```python
from build123d import *

# Parameters (mm, degrees)
STEM_START                = 6.825155764
STEM_OTHER_SIDE_OUTLINE_W = 12.827
STEM_OTHER_SIDE_OUTLINE_H = 3.302
STEM_OTHER_SIDE_OUTLINE_R = 3.81
STEM_OTHER_SIDE_DEPTH     = 3.175
SKETCH2_R                 = 1.5875
CUT_EXTRUDE1_DEPTH        = 3.175
FILLET1_R                 = 8.89
FILLET2_R                 = 8.89


# Read off the part's stored shape, not the designer's step: Stem Other Side
with BuildPart() as part:
    # Stem Other Side outline → Stem Other Side (new body)
    with BuildSketch(Plane(origin=(0, 0, 0), x_dir=(1, 0, 0), z_dir=(0, 1, 0)).offset(STEM_START)):
        with BuildLine():
            Line((-15.619811821, 34.159467437), (-16.889811821, 34.159467437))
            ThreePointArc((-16.889811821, 34.159467437), (-23.175991106, 31.555646722), (-25.779811821, 25.269467437))
            Line((-25.779811821, 25.269467437), (-25.779811821, -42.040532563))
            Line((-25.779811821, -42.040532563), (-6.729811821, -42.040532563))
            Line((-6.729811821, -42.040532563), (-6.729811821, 25.269467437))
            ThreePointArc((-6.729811821, 25.269467437), (-9.333632536, 31.555646722), (-15.619811821, 34.159467437))
        make_face()
        with Locations((-16.254811821, -11.941532563)):
            Rectangle(STEM_OTHER_SIDE_OUTLINE_W, STEM_OTHER_SIDE_OUTLINE_H, mode=Mode.SUBTRACT)
        with Locations((-16.254811821, 21.459467437)):
            Circle(STEM_OTHER_SIDE_OUTLINE_R, mode=Mode.SUBTRACT)
    extrude(amount=STEM_OTHER_SIDE_DEPTH)

    # Sketch2 → Cut-Extrude1 (cut)
    with BuildSketch(Plane(origin=(0, 10.000155764, 0), x_dir=(1, 0, 0), z_dir=(0, 1, 0))):
        with Locations(Location((-16.254811821, -29.340532563, 0), (0, 0, 270))):
            Circle(SKETCH2_R)
    extrude(amount=-CUT_EXTRUDE1_DEPTH, mode=Mode.SUBTRACT)

    # Fillet1
    fillet1_edges = [part.edges().sort_by_distance(p)[0] for p in [
        (-6.729811821, 8.412655764, 42.040532563),
    ]]
    fillet(fillet1_edges, radius=FILLET1_R)

    # Fillet2
    fillet2_edges = [part.edges().sort_by_distance(p)[0] for p in [
        (-25.779811821, 8.412655764, 42.040532563),
    ]]
    fillet(fillet2_edges, radius=FILLET2_R)


solid = part.part
```
Can you work these out from the model? Positions are in its coordinate system, mm. A direction names the side the tool comes from. Round coordinates to 2 decimals unless told otherwise and drop trailing zeros. Loops run counter-clockwise (first coordinate to the right, second up) from the corner with the lowest first, then second, coordinate; pieces in that order, holes last.
Item 1: Please list where these lines run through material, in increasing order: L1, parallel to Z at x = -18.25, y = 8.4; L2, parallel to Z at x = -17.5, y = 8.7; L3, parallel to X at y = 8.7, z = -22.5.
Item 2: Suppose I cut it at C-C, the plane z = -27.5. Write out the boundary of the cut face in (x, y).
Item 3: Which directions (+Z, -Z, +X, -X, +Y, -Y) give clear straight access to the entire face, cutting with the end or side of a thin tool? Please do faces 4 (the flat face through (-16, 8, 10.291)), 5 (the flat face through (-16, 10, 3)).
Item 4: Will this pin go through, and if not, where does the flat tip stop? pin 1 Ø5 at (x, z) = (-16.25, 29.34) entering from +Y.
Item 5: Suppose I cut it at A-A, the plane y = 9.3. Write out the boundary of the cut face in (x, z) (1 decimal), then the cut area to 3 significant figures.
Item 6: Suppose I cut it at B-B, the plane z = 35.5. Write out the boundary of the cut face in (x, y).
Item 7: If we mould it in two halves opening along Z, with no side actions, what happens to faces 1 (the cylindrical face through (-9.265, 8.435, 39.367)), 2 (the flat face through (-25.78, 8, 4)), 3 (the flat face through (-9.841, 8, 12))? For each: +Z half, -Z half, draft (parallel to the pull), parting line (faces both ways), or undercut.
Reported:
1. L1: z = -34.05 to -24.71, -18.21 to 10.29, 13.59 to 41.94
1. L2: z = -34.14 to -25.06, -17.86 to 10.29, 13.59 to 28.36, 30.33 to 42.02
1. L3: x = -25.78 to -19.92, -12.59 to -6.73
2. outline: (-25.5, 6.83) - (-7.01, 6.83) - (-7.01, 10) - (-25.5, 10) - close
3. face 4: +Y, -Y
3. face 5: +Z, -Z, +X, -X, +Y
4. pin 1: stops at y = 10
5. outline: (-25.8, -25.3) arc R8.9 ccw to (-16.9, -34.2) - (-15.6, -34.2) arc R8.9 ccw to (-6.7, -25.3) - (-6.7, 33.2) arc R8.9 ccw to (-15.6, 42) - (-16.9, 42) arc R8.9 ccw to (-25.8, 33.2) - close; hole (-22.7, 10.3) - (-9.8, 10.3) - (-9.8, 13.6) - (-22.7, 13.6) - close; hole circle Ø7.6 at (-16.3, -21.5); hole circle Ø3.2 at (-16.3, 29.3)
5. area: 1,290 mm2
6. outline: (-25.46, 6.83) - (-7.05, 6.83) - (-7.05, 10) - (-25.46, 10) - close
7. face 1: +Z half
7. face 2: draft
7. face 3: undercut
